Verification items for the finished model (mm, model axes). A direction names the side the tool comes from. Give positions to 0.01 mm unless a question says otherwise; leave off trailing zeros. Order: outer loops, then holes, each group sorted by start corner. A loop starts at its lowest first (then second) coordinate and runs counter-clockwise, first axis right, second up. Notation, with made-up numbers: (22, 47.5) -> (73, 47.5) arc R13 ccw to (73, 67.5) -> close; hole circle Ø6 at (1.5, 56). An arc over 180 degrees is marked (long way). Return JSON: item names as keys, results as strings. Group by question number.
(1) Cross-section at C-C on y = 5.5. Enter the section's corners in (x, z), then the cut area to 3 significant figures.
(2) Thickness scan on line 1 along X through (y, z) = (15.5, 0) (3 decimals); line 2 along Z through (x, y) = (-11.5, 14.25); line 3 along X through (y, z) = (6.25, -3.75). Record the ranges inside material, lowest first.
(3) Release check for a two-part mould opening along X. For faces 5 (the face through (13.5, 7, -6)), 6 (the face through (5, 16, 7)), 7 (the face through (0, 8, 6.25)) record: pulls with the +X half, pulls with the -X half, needs draft (parallel to the pull), parting line crosses it, or undercut.
(4) Cross-section at D-D on y = 14.5. Enter the section's corners in (x, z) (3 decimals), then the cut area to 3 significant figures.
(5) Depth check by flat-ended pin: pin 1 Ø3.5 at (y, z) = (4, 6.5) entering from +X; pin 2 Ø1.6 at (x, z) = (13.625, 0) entering from -Y; pin 3 Ø0.9 at (x, z) = (-13, 0) entering from +Y. Enter the tip coordinate at first touch or a pass-through.
(6) Tool access check on faces 1 (the face through (13, 7, 3.5)), 2 (the face through (-13, 3, 0)), 3 (the face through (13.5, 7, 6)), 4 (the face through (-11.75, 6, 3)). Record the directions out of +Z, -Z, +X, -X, +Y, -Y that give a thin tool (end or side, any length) a straight path to the whole face; none if there is none.
(7) Cross-section at B-B on x = 5.5. Enter the section's corners in (y, z), then the cut area to 3 significant figures.
(8) Cross-section at A-A on z = -1.75. Enter the section's corners in (x, y), then the cut area to 4 significant figures.
from build123d import *

# Parameters (mm, degrees)
SKETCH1_W           = 27
SKETCH1_H           = 16
BOSS_EXTRUDE1_DEPTH = 16
SKETCH2_W           = 23.5
SKETCH2_H           = 12.5
CUT_EXTRUDE1_DEPTH  = 16
SKETCH3_W           = 5.5
SKETCH3_H           = 13
CUT_EXTRUDE2_DEPTH  = 4
SKETCH4_W           = 16
SKETCH4_H           = 2
BOSS_EXTRUDE2_DEPTH = 4
SKETCH5_R           = 1
CUT_EXTRUDE3_DEPTH  = 17
SKETCH6_W           = 7
SKETCH6_H           = 14
CUT_EXTRUDE4_DEPTH  = 4


with BuildPart() as part:
    # Sketch1 → Boss-Extrude1 (new body)
    with BuildSketch(Plane(origin=(0, 0, 0), x_dir=(1, 0, 0), z_dir=(0, 1, 0))):
        Rectangle(SKETCH1_W, SKETCH1_H)
    extrude(amount=BOSS_EXTRUDE1_DEPTH)

    # Sketch2 → Cut-Extrude1 (cut)
    with BuildSketch(Plane(origin=(0, 16, 0), x_dir=(1, 0, 0), z_dir=(0, 1, 0))):
        Rectangle(SKETCH2_W, SKETCH2_H)
    extrude(amount=-CUT_EXTRUDE1_DEPTH, mode=Mode.SUBTRACT)

    # Sketch3 → Cut-Extrude2 (cut)
    with BuildSketch(Plane.ZY.offset(13.5)):
        with Locations((0, 9.5)):
            Rectangle(SKETCH3_W, SKETCH3_H)
    extrude(amount=-CUT_EXTRUDE2_DEPTH, mode=Mode.SUBTRACT)

    # Sketch4 → Boss-Extrude2 (add)
    with BuildSketch(Plane(origin=(13.5, 0, 0), x_dir=(0, 0, -1), z_dir=(1, 0, 0))):
        with Locations((0, 15)):
            Rectangle(SKETCH4_W, SKETCH4_H)
    extrude(amount=BOSS_EXTRUDE2_DEPTH)

    # Sketch5 → Cut-Extrude3 (cut, through all)
    with BuildSketch(Plane(origin=(0, 16, 0), x_dir=(1, 0, 0), z_dir=(0, 1, 0))):
        with Locations((13.625, 0)):
            Circle(SKETCH5_R)
    extrude(amount=-CUT_EXTRUDE3_DEPTH, mode=Mode.SUBTRACT)

    # Sketch6 → Cut-Extrude4 (cut)
    with BuildSketch(Plane(origin=(13.5, 0, 0), x_dir=(0, 0, -1), z_dir=(1, 0, 0))):
        with Locations((0, 7)):
            Rectangle(SKETCH6_W, SKETCH6_H)
    extrude(amount=-CUT_EXTRUDE4_DEPTH, mode=Mode.SUBTRACT)


solid = part.part
Verdict:
{
 "1": {"outline": "(-13.5, -8) -> (13.5, -8) -> (13.5, -3.5) -> (11.75, -3.5) -> (11.75, -6.25) -> (-11.75, -6.25) -> (-11.75, -2.75) -> (-13.5, -2.75) -> close; (-13.5, 2.75) -> (-11.75, 2.75) -> (-11.75, 6.25) -> (11.75, 6.25) -> (11.75, 3.5) -> (13.5, 3.5) -> (13.5, 8) -> (-13.5, 8) -> close", "area": "116 mm²"},
 "2": {"line 1": "11.75 to 12.625, 14.625 to 17.5", "line 2": "-8 to -6.25, 6.25 to 8", "line 3": "-13.5 to -11.75, 11.75 to 13.5"},
 "3": {"face 5": "pulls with the +X half", "face 6": "needs draft", "face 7": "undercut"},
 "4": {"outline": "(-13.5, -8) -> (17.5, -8) -> (17.5, 8) -> (-13.5, 8) -> (-13.5, 2.75) -> (-11.75, 2.75) -> (-11.75, 6.25) -> (11.75, 6.25) -> (11.75, -6.25) -> (-11.75, -6.25) -> (-11.75, -2.75) -> (-13.5, -2.75) -> close; hole circle Ø2 at (13.625, 0)", "area": "189 mm²"},
 "5": {"pin 1": "x = 13.5", "pin 2": "through", "pin 3": "y = 3"},
 "6": {"face 1": "+X, -Y", "face 2": "+X, -X, +Y", "face 3": "+Z, -Z, +X, -Y", "face 4": "+Y, -Y"},
 "7": {"outline": "(0, -8) -> (16, -8) -> (16, -6.25) -> (0, -6.25) -> close; (0, 6.25) -> (16, 6.25) -> (16, 8) -> (0, 8) -> close", "area": "56.0 mm²"},
 "8": {"outline": "(-13.5, 0) -> (-11.75, 0) -> (-11.75, 3) -> (-13.5, 3) -> close; (11.75, 14) -> (17.5, 14) -> (17.5, 16) -> (11.75, 16) -> close", "area": "16.75 mm²"}
}
